For this review, take the finished solid that the model builds, in its own axes (mm). Face numbers are marked on the shaded views. Give positions to 0.01 mm unless a question says otherwise; leave off trailing zeros. Order: outer loops, then holes, each group sorted by start corner. A loop starts at its lowest first (then second) coordinate and runs counter-clockwise, first axis right, second up.
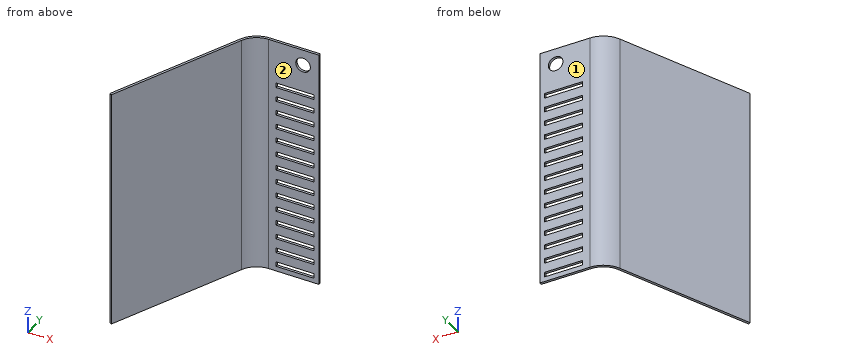
from build123d import *

# Parameters (mm, degrees)
EXTRUDE_THIN1_DEPTH = 500
SKETCH3_W           = 155.92
SKETCH3_H           = 20
CUT_EXTRUDE1_DEPTH  = 226
LPATTERN1_COUNT     = 14
LPATTERN1_PITCH     = 60
SKETCH4_R           = 30
CUT_EXTRUDE2_DEPTH  = 226


with BuildPart() as part:
    # Sketch1 → Extrude-Thin1 (new, symmetric)
    with BuildSketch(Plane.XY):
        with BuildLine():
            Line((0, 0), (-205.92, 0))
            ThreePointArc((-205.92, 0), (-259.855879639, -15.792394123), (-296.756225905, -58.181582248))
            Line((-296.756225905, -58.181582248), (-539.303048865, -585.0316925))
            Line((-539.303048865, -585.0316925), (-530.219426274, -589.213534275))
            Line((-530.219426274, -589.213534275), (-287.672603315, -62.363424024))
            ThreePointArc((-287.672603315, -62.363424024), (-254.462291675, -24.21315471), (-205.92, -10))
            Line((-205.92, -10), (0, -10))
            Line((0, -10), (0, 0))
        make_face()
    extrude(amount=EXTRUDE_THIN1_DEPTH, both=True)

    # Sketch3 → Cut-Extrude1 (cut, symmetric)
    with BuildSketch(Plane(origin=(0, 0, 0), x_dir=(1, 0, 0), z_dir=(0, 1, 0))):
        with Locations((-97.96, 470)):
            Rectangle(SKETCH3_W, SKETCH3_H)
    cut_extrude1 = extrude(amount=CUT_EXTRUDE1_DEPTH, both=True, mode=Mode.SUBTRACT)

    # LPattern1: Cut-Extrude1 ×14
    with Locations(*[(0, 0, i * LPATTERN1_PITCH) for i in range(1, LPATTERN1_COUNT)]):
        add(cut_extrude1, mode=Mode.SUBTRACT)

    # Sketch4 → Cut-Extrude2 (cut, symmetric)
    with BuildSketch(Plane(origin=(0, 0, 0), x_dir=(1, 0, 0), z_dir=(0, 1, 0))):
        with Locations(Location((-65, -435, 0), (0, 0, 180))):
            Circle(SKETCH4_R)
    extrude(amount=CUT_EXTRUDE2_DEPTH, both=True, mode=Mode.SUBTRACT)


solid = part.part
1) To check wall thickness, follow line 1 (Y direction, x = -35, z = -151); line 2 (Y direction, x = -337, z = 191); line 3 (X direction, y = -474, z = 392). State the ranges of each line that lie inside material, in increasing order.
Answer sheet:
line 1: y = -10 to 0
line 2: y = -169.51 to -145.6
line 3: x = -488.19 to -477.18
2) We need section A-A on z = 435. Give the boundary of the cut face in (x, y).
Answer sheet:
outline: (-539.3, -585.03) - (-530.22, -589.21) - (-287.67, -62.36) arc R90 cw to (-205.92, -10) - (-95, -10) - (-95, 0) - (-205.92, 0) arc R100 ccw to (-296.76, -58.18) - close; (-35, -10) - (0, -10) - (0, 0) - (-35, 0) - close
3) Clearance check with flat-ended pins moving along their axes: pin 1 (8 mm diameter, centred on y = -5, z = -169, fed in from +X); pin 2 (2 mm diameter, centred on x = -76.5, z = -197, fed in from -Y); pin 3 (5 mm diameter, centred on y = -6, z = 131.5, fed in from -X); pin 4 (10 mm diameter, centred on y = -480, z = 62.5, fed in from -X). State where each tip first meets the part, or that it passes through.
Answer sheet:
pin 1: stops at x = 0
pin 2: stops at y = -10
pin 3: stops at x = -246.27
pin 4: stops at x = -493.25
4) We need section C-C on x = -65. Count the separate pieces of the cut face and the enclosed holes in it, then the cut area to 3 significant figures.
Answer sheet:
separate pieces: 16
enclosed holes: 0
area: 6,600 mm2
5) We need section B-B on z = 44. Give the boundary of the cut face in (x, y), then the cut area to 3 significant figures.
Answer sheet:
outline: (-539.3, -585.03) - (-530.22, -589.21) - (-287.67, -62.36) arc R90 cw to (-205.92, -10) - (0, -10) - (0, 0) - (-205.92, 0) arc R100 ccw to (-296.76, -58.18) - close
area: 8,940 mm2
6) Draft analysis for pull direction Y (two halves, no side actions). For the marked faces 1 and 2, state which applies: +Y half, -Y half, draft (parallel to the pull), parting line (faces both ways), or undercut.
Answer sheet:
face 1: +Y half
face 2: -Y half
7) We need section D-D on y = -531. Give the boundary of the cut face in (x, z).
Answer sheet:
outline: (-514.43, -500) - (-503.42, -500) - (-503.42, 500) - (-514.43, 500) - close
